For this review, take the finished solid that the model builds, in its own axes (mm). A direction names the side the tool comes from. Round coordinates to 2 decimals unless told otherwise and drop trailing zeros. Write each loop counter-clockwise with the first axis right and the second up, starting at its lowest first coordinate (ties: lowest second). Pieces come first, ordered by that corner, then holes. Notation, with made-up numbers: M 86.25,-6 L 131.25,-6 A32 cw 131.25,25 Z; hole C 82.25,34.5 d10. An arc over 180 degrees is marked long. Answer in a Markdown table with one row per item.
```python
from build123d import *

# Parameters (mm, degrees)
F0_W     = 64
F0_H     = 38
F0_R     = 1.5875
F0_R_2   = 5.1
F1_DEPTH = 3
F0_H_2   = 4
F2_DEPTH = 32
F3_R     = 12.7
F4_R     = 1.5875
F5_DEPTH = 4
F6_R     = 1.27
F7_R     = 0.8
F8_R     = 1.27


with BuildPart() as f1:
    # F0 (on Front) → F1 (new body)
    with BuildSketch(Plane.XZ):
        with Locations((32, 19)):
            Rectangle(F0_W, F0_H)
        with Locations((16, 19)):
            Circle(F0_R, mode=Mode.SUBTRACT)
        with Locations((32, 19)):
            Circle(F0_R_2, mode=Mode.SUBTRACT)
        with Locations((48, 19)):
            Circle(F0_R, mode=Mode.SUBTRACT)
    extrude(amount=F1_DEPTH)

    # F0 (on Front) → F2 (join)
    with BuildSketch(Plane.XZ):
        with Locations((32, 40)):
            Rectangle(F0_W, F0_H_2)
        with Locations((32, -2)):
            Rectangle(F0_W, F0_H_2)
    extrude(amount=F2_DEPTH)

    # F3
    f3_edges = [f1.edges().sort_by_distance(p)[0] for p in [
        (64, -32, -2),
        (64, -32, 40),
        (0, -32, -2),
        (0, -32, 40),
    ]]
    fillet(f3_edges, radius=F3_R)

    # F4 (on face) → F5 (cut, through all)
    with BuildSketch(Plane(origin=(0, 0, -4), x_dir=(1, 0, 0), z_dir=(0, 0, -1))):
        with Locations((48, 16)):
            Circle(F4_R)
        with Locations((32, 24)):
            Circle(F4_R)
        with Locations((32, 16)):
            Circle(F4_R)
        with Locations((32, 8)):
            Circle(F4_R)
        with Locations((16, 16)):
            Circle(F4_R)
    extrude(amount=-F5_DEPTH, mode=Mode.SUBTRACT)

    # F6
    f6_edges = [f1.edges().sort_by_distance(p)[0] for p in [
        (0, -11.15, 38),
        (0, -9.65, 42),
        (0, -9.65, -4),
        (0, -11.15, 0),
        (0, -3, 19),
        (64, -3, 19),
    ]]
    fillet(f6_edges, radius=F6_R)

    # F7
    f7_edges = [f1.edges().sort_by_distance(p)[0] for p in [
        (26.9, 0, 19),
    ]]
    fillet(f7_edges, radius=F7_R)

    # F8
    f8_edges = [f1.edges().sort_by_distance(p)[0] for p in [
        (32, 0, -4),
        (32, 0, 42),
    ]]
    fillet(f8_edges, radius=F8_R)


solid = f1.part
```
Q1. Take a section at C-C (y = -16). State the section outline as (x, z) points.
Found:
| item | result |
|---|---|
| outline | M 0,-2.73 A1.27 ccw 1.27,-4 L 14.41,-4 L 14.41,0 L 1.27,0 A1.27 ccw 0,-1.27 Z; M 0,39.27 A1.27 ccw 1.27,38 L 62.73,38 A1.27 ccw 64,39.27 L 64,40.73 A1.27 ccw 62.73,42 L 1.27,42 A1.27 ccw 0,40.73 Z; M 17.59,-4 L 30.41,-4 L 30.41,0 L 17.59,0 Z; M 33.59,-4 L 46.41,-4 L 46.41,0 L 33.59,0 Z; M 49.59,-4 L 62.73,-4 A1.27 ccw 64,-2.73 L 64,-1.27 A1.27 ccw 62.73,0 L 49.59,0 Z |
Q2. Machinability: for faces 5 (the face through (15.66, -14.45, -2.03)), 6 (the face through (32, -14, 0)), 7 (the face through (32, -16, 42)), which of the approach directions +Z, -Z, +X, -X, +Y, -Y give a long, thin tool a straight path to every point of the face, cutting with its end or side? Answer none if there is none.
Found:
| item | result |
|---|---|
| face 5 | -Z |
| face 6 | +X, -X, -Y |
| face 7 | +Z, +X, -X, +Y, -Y |
Q3. For probe 1 along Y at (x, z) = (32, -1.5); probe 2 along X at (y, z) = (-16, -2); probe 3 along Z at (x, y) = (6.5, -6), list the stretches that pass through material, from the lowest coordinate up.
Found:
| item | result |
|---|---|
| probe 1 | -32 to -25.59, -22.41 to -17.59, -14.41 to -9.59, -6.41 to 0 |
| probe 2 | 0 to 14.41, 17.59 to 30.41, 33.59 to 46.41, 49.59 to 64 |
| probe 3 | -4 to 0, 38 to 42 |
Q4. Take a section at D-D (z = 3). State the section outline as (x, y) points.
Found:
| item | result |
|---|---|
| outline | M 0,-1.73 A1.27 ccw 1.27,-3 L 62.73,-3 A1.27 ccw 64,-1.73 L 64,-1.27 A1.27 ccw 62.73,0 L 1.27,0 A1.27 ccw 0,-1.27 Z |
Q5. Take a section at B-B (y = -8). State the section outline as (x, z) points.
Found:
| item | result |
|---|---|
| outline | M 0,-2.73 A1.27 ccw 1.27,-4 L 30.41,-4 L 30.41,0 L 1.27,0 A1.27 ccw 0,-1.27 Z; M 0,39.27 A1.27 ccw 1.27,38 L 62.73,38 A1.27 ccw 64,39.27 L 64,40.73 A1.27 ccw 62.73,42 L 1.27,42 A1.27 ccw 0,40.73 Z; M 33.59,-4 L 62.73,-4 A1.27 ccw 64,-2.73 L 64,-1.27 A1.27 ccw 62.73,0 L 33.59,0 Z |
Q6. Insertion check: P1, Ø11.5, axis at x = 32.5, z = 16, coming from the -Y side. The pin has a flat end and moves straight along its axis. Give the tip position at first contact, or say it passes through.
Found:
| item | result |
|---|---|
| P1 | y = -3 |
Q7. Mouldability with a two-part tool opening along Z and no side actions: class faces 1 (the face through (32, -13, -4)), 2 (the face through (32, -17, 38)), 3 (the face through (32, -32, -2)), 4 (the face through (15.66, -1.48, 17.45)) as +Z half, -Z half, draft (parallel to the pull), parting line (faces both ways), or undercut.
Found:
| item | result |
|---|---|
| face 1 | -Z half |
| face 2 | undercut |
| face 3 | draft |
| face 4 | undercut |
Q8. Take a section at A-A (x = 48). State the section outline as (y, z) points, then the cut area to 3 significant figures.
Found:
| item | result |
|---|---|
| outline | M -32,-2.73 A1.27 ccw -30.73,-4 L -17.59,-4 L -17.59,0 L -30.73,0 A1.27 ccw -32,-1.27 Z; M -32,39.27 A1.27 ccw -30.73,38 L -3,38 L -3,20.59 L 0,20.59 L 0,40.73 A1.27 ccw -1.27,42 L -30.73,42 A1.27 ccw -32,40.73 Z; M -14.41,-4 L -1.27,-4 A1.27 ccw 0,-2.73 L 0,17.41 L -3,17.41 L -3,0 L -14.41,0 Z |
| area | 346 mm² |
